from build123d import *

# Parameters (mm, degrees)
F0_W      = 10
F0_H      = 10
F1_DEPTH  = 150
F3_D      = 2.5
F3_DEPTH  = 15
F3_TIP    = 0.7510757738
F5_D      = 2.5
F5_DEPTH  = 15
F5_TIP    = 0.7510757738
F7_D      = 2.5
F7_DEPTH  = 10
F7_TIP    = 0.7510757738
F9_D      = 2.5
F9_DEPTH  = 10
F9_TIP    = 0.7510757738
F11_D     = 2.5
F11_DEPTH = 10
F11_TIP   = 0.7510757738
F13_D     = 2.5
F13_DEPTH = 10
F13_TIP   = 0.7510757738
F15_D     = 2.5
F15_DEPTH = 10
F15_TIP   = 0.7510757738
F17_D     = 2.5
F17_DEPTH = 10
F17_TIP   = 0.7510757738
F19_D     = 2.5
F19_DEPTH = 10
F19_TIP   = 0.7510757738


with BuildPart() as f1:
    # F0 (on Top) → F1 (new body)
    with BuildSketch(Plane.XY):
        with Locations((5, -5)):
            Rectangle(F0_W, F0_H)
    extrude(amount=F1_DEPTH)

    # F3
    with Locations(Plane.XY.offset(150)):
        with Locations((5, -5)):
            Hole(F3_D / 2, depth=F3_DEPTH)
            with Locations((0, 0, -(F3_DEPTH + F3_TIP / 2))):  # 118° drill point
                Cone(0, F3_D / 2, F3_TIP, mode=Mode.SUBTRACT)

    # F5
    with Locations(Plane(origin=(0, 0, 0), x_dir=(1, 0, 0), z_dir=(0, 0, -1))):
        with Locations((5, 5.128350097)):
            Hole(F5_D / 2, depth=F5_DEPTH)
            with Locations((0, 0, -(F5_DEPTH + F5_TIP / 2))):  # 118° drill point
                Cone(0, F5_D / 2, F5_TIP, mode=Mode.SUBTRACT)

    # F7
    with Locations(Plane(origin=(0, 0, 0), x_dir=(-1, 0, 0), z_dir=(0, 1, 0))):
        with Locations((-5, 5)):
            Hole(F7_D / 2, depth=F7_DEPTH)
            with Locations((0, 0, -(F7_DEPTH + F7_TIP / 2))):  # 118° drill point
                Cone(0, F7_D / 2, F7_TIP, mode=Mode.SUBTRACT)

    # F9
    with Locations(Plane.XZ.offset(10)):
        with Locations((5.0156186335, 145)):
            Hole(F9_D / 2, depth=F9_DEPTH)
            with Locations((0, 0, -(F9_DEPTH + F9_TIP / 2))):  # 118° drill point
                Cone(0, F9_D / 2, F9_TIP, mode=Mode.SUBTRACT)

    # F11
    with Locations(Plane.XZ.offset(10)):
        with Locations((5, 65)):
            Hole(F11_D / 2, depth=F11_DEPTH)
            with Locations((0, 0, -(F11_DEPTH + F11_TIP / 2))):  # 118° drill point
                Cone(0, F11_D / 2, F11_TIP, mode=Mode.SUBTRACT)

    # F13
    with Locations(Plane.XZ.offset(10)):
        with Locations((5, 105)):
            Hole(F13_D / 2, depth=F13_DEPTH)
            with Locations((0, 0, -(F13_DEPTH + F13_TIP / 2))):  # 118° drill point
                Cone(0, F13_D / 2, F13_TIP, mode=Mode.SUBTRACT)

    # F15
    with Locations(Plane.YZ.offset(10)):
        with Locations((-5, 145)):
            Hole(F15_D / 2, depth=F15_DEPTH)
            with Locations((0, 0, -(F15_DEPTH + F15_TIP / 2))):  # 118° drill point
                Cone(0, F15_D / 2, F15_TIP, mode=Mode.SUBTRACT)

    # F17
    with Locations(Plane.YZ.offset(10)):
        with Locations((-5, 5)):
            Hole(F17_D / 2, depth=F17_DEPTH)
            with Locations((0, 0, -(F17_DEPTH + F17_TIP / 2))):  # 118° drill point
                Cone(0, F17_D / 2, F17_TIP, mode=Mode.SUBTRACT)

    # F19
    with Locations(Plane.YZ.offset(10)):
        with Locations((-5, 85)):
            Hole(F19_D / 2, depth=F19_DEPTH)
            with Locations((0, 0, -(F19_DEPTH + F19_TIP / 2))):  # 118° drill point
                Cone(0, F19_D / 2, F19_TIP, mode=Mode.SUBTRACT)


solid = f1.part
Geometry check sheet. Reference: the model listing, model coordinates, mm. A direction names the side the tool comes from. Round coordinates to 2 decimals unless told otherwise and drop trailing zeros. Order: outer loops, then holes, each group sorted by start corner. A loop starts at its lowest first (then second) coordinate and runs counter-clockwise, first axis right, second up. Notation, with made-up numbers: M -30,43 L 11,43 A24 ccw 11,68 Z; hole C 81.5,81 d10. An arc over 180 degrees is marked long. Answer in a Markdown table with one row per item. Add a question column.
Item 1: Sectioned sample at B-B, the plane z = 136.5. Enter the section's corners in (x, y).
Item 2: Sectioned sample at A-A, the plane z = 65. Enter the section's corners in (x, y).
Item 3: Material ranges on L1, parallel to Z at x = 3.5, y = -5; L2, parallel to X at y = -3.1, z = 5; L3, parallel to Z at x = 7, y = -4, recorded low to high. Write a range as [from, to].
Item 4: Draft check along Y on faces 4 (the face through (5.921, -5.973, 2.121)), 5 (the face through (5, 0, 74)), 6 (the face through (0, -5, 74)). Enter one of: released by +Y, released by -Y, zero draft, split by the parting line, or undercut.
Item 5: Depth check by flat-ended pin: pin 1 Ø2 at (y, z) = (-5, 145) entering from -X. Enter the tip coordinate at first touch or a pass-through.
Item 6: Set-up check for faces 1 (the face through (6.25, -5.18, 10.47)), 2 (the face through (5.921, -4.155, 147.909)), 3 (the face through (5, -10, 74)): record each of +Z, -Z, +X, -X, +Y, -Y from which the full face is reachable in a straight line by a thin tool's end or side.
Filled in:
| question | item | result |
|---|---|---|
| 1 | outline | M 0,-10 L 10,-10 L 10,0 L 0,0 Z; hole C 5,-5 d2.5 |
| 2 | outline | M 0,-10 L 3.75,-10 L 3.75,0 L 0,0 Z; M 6.25,-10 L 10,-10 L 10,0 L 6.25,0 Z |
| 3 | L1 | z = [0, 3.75], [6.25, 83.75], [86.25, 143.75], [146.25, 150] |
| 3 | L2 | x = [0, 3.75], [6.25, 10] |
| 3 | L3 | z = [0, 4.25], [5.75, 84.25], [85.75, 144.25], [145.75, 150] |
| 4 | face 4 | undercut |
| 4 | face 5 | released by +Y |
| 4 | face 6 | zero draft |
| 5 | pin 1 | passes through |
| 6 | face 1 | -Z |
| 6 | face 2 | +Z |
| 6 | face 3 | +Z, -Z, +X, -X, -Y |
